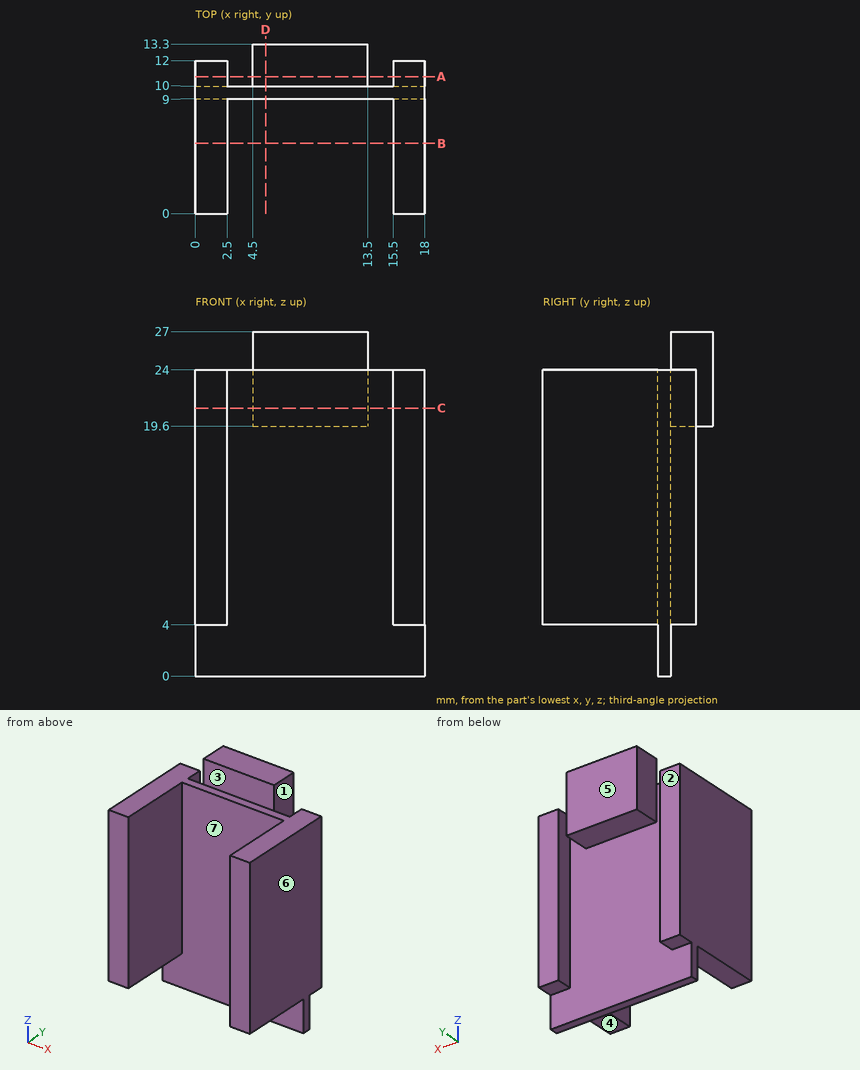
Source: three-view drawing plus pictorial views. Frame: mm from the lowest corner of the part. A direction names the side the tool comes from. Coordinates: 2 decimals unless noted, no trailing zeros. Order: outer loops, then holes, each group sorted by start corner. A loop starts at its lowest first (then second) coordinate and runs counter-clockwise, first axis right, second up.
Item 1: Cut plane C-C (z = 21). Return loops of the section in (x, y).
Output values:
outline: (0, 0) - (2.5, 0) - (2.5, 9) - (15.5, 9) - (15.5, 0) - (18, 0) - (18, 12) - (15.5, 12) - (15.5, 10) - (13.5, 10) - (13.5, 13.3) - (4.5, 13.3) - (4.5, 10) - (2.5, 10) - (2.5, 12) - (0, 12) - close
Item 2: First-contact query: P1, Ø2, axis at x = 9, y = 8.5, coming from the -Z side; P2, Ø4, axis at x = 15.5, y = 9, coming from the +Z side; P3, Ø2.5, axis at x = 9.5, z = 25.5, coming from the -Y side; P4, Ø3, axis at x = 6, z = 3, coming from the -Y side. Flat tips, straight axial feed; report the tip coordinate or a pass-through.
Output values:
P1: stops at z = 0
P2: stops at z = 24
P3: stops at y = 10
P4: stops at y = 9
Item 3: Pull-direction query (X, two-part tool) for the marked faces 5, 6 and 7; classes: pulls with the +X half, pulls with the -X half, needs draft (parallel to the pull), parting line crosses it, or undercut.
Output values:
face 5: needs draft
face 6: pulls with the +X half
face 7: undercut
Item 4: Material intervals for line 1 (X direction, y = 1, z = 22.75); line 2 (Z direction, x = 16, y = 3); line 3 (Y direction, x = 10, z = 9), sorted ascending.
Output values:
line 1: x = 0 to 2.5, 15.5 to 18
line 2: z = 4 to 24
line 3: y = 9 to 10
Item 5: Cut plane B-B (y = 5.5). Return loops of the section in (x, z).
Output values:
outline: (0, 4) - (2.5, 4) - (2.5, 24) - (0, 24) - close; (15.5, 4) - (18, 4) - (18, 24) - (15.5, 24) - close
Item 6: Cut plane D-D (x = 5.5). Return loops of the section in (y, z).
Output values:
outline: (9, 0) - (10, 0) - (10, 19.6) - (13.3, 19.6) - (13.3, 27) - (10, 27) - (10, 24) - (9, 24) - close
Item 7: Set-up query: the marked faces 1, 2, 3 and 4. Return all of +Z, -Z, +X, -X, +Y, -Y with unobstructed straight access to the full face (end or side cutting, diameter ignored); none if empty.
Output values:
face 1: +Z, -Z, +Y
face 2: +Z, -Z, -X, +Y
face 3: +Z, +X, -X, -Y
face 4: -Z, +X, -X, -Y
Item 8: Cut plane A-A (y = 10.75). Return loops of the section in (x, z).
Output values:
outline: (0, 4) - (2.5, 4) - (2.5, 24) - (0, 24) - close; (4.5, 19.6) - (13.5, 19.6) - (13.5, 27) - (4.5, 27) - close; (15.5, 4) - (18, 4) - (18, 24) - (15.5, 24) - close
